Source: CAD feature listing. Evaluate the final solid. Frame: model axes, mm. Coordinates: 2 decimals unless noted, no trailing zeros. Order: outer loops, then holes, each group sorted by start corner. A loop starts at its lowest first (then second) coordinate and runs counter-clockwise, first axis right, second up. Notation, with made-up numbers: (-28.5, 4) - (-16.5, 4) arc R16 ccw to (-16.5, 24) - close; hole circle Ø6 at (20.5, -8). An arc over 180 degrees is marked (long way). One line per question, with ' | ' between items. Start each with the question number.
(1) Section D-D (x = 30). Return the cut outline in (y, z), then the cut area to 3 significant figures.
(2) Section C-C (y = -53). Return the cut outline in (x, z), then the cut area to 3 significant figures.
(3) Section B-B (y = -9). Return the cut outline in (x, z).
(4) Draft query along Y for faces 1 (the cylindrical face through (98.052, -41.158, 0.739)), 2 (the flat face through (58, -37, 0)), 3 (the flat face through (8, -93, 1)), 4 (the flat face through (8, -5, 1)). Return one class per face: +Y half, -Y half, draft (parallel to the pull), parting line (faces both ways), or undercut.
(5) Section A-A (x = 12.5). Return the cut outline in (y, z), then the cut area to 3 significant figures.
(6) Line query: line 1 along Y through (x, z) = (30, 1.1); line 2 along X through (y, z) = (-84, 0.6); line 3 along Y through (x, z) = (36.5, 1.1). Output: solid intervals per line, ascending.
from build123d import *

# Parameters (mm, degrees)
BOSS_EXTRU_1_DEPTH      = 1.5
ESQUISSE2_R             = 1.5
ESQUISSE2_W             = 14
ESQUISSE2_H             = 14
ENL_V_MAT_EXTRU_1_DEPTH = 1.5
D_GAGEMENT_M31_D        = 3.6


with BuildPart() as part:
    # Esquisse1 → Boss.-Extru.1 (new body)
    with BuildSketch(Plane.XY):
        Polygon((0, -85), (16, -101), (117.25, -101), (117.25, 3), (16, 3), (0, -13), align=None)
    extrude(amount=BOSS_EXTRU_1_DEPTH)

    # Esquisse2 → Enlèv. mat.-Extru.1 (cut)
    with BuildSketch(Plane.XY.offset(1.5)):
        with Locations((30, -9)):
            Circle(ESQUISSE2_R)
        with Locations((11, -32.85)):
            Rectangle(ESQUISSE2_W, ESQUISSE2_H)
        with Locations((30.05, -32.85)):
            Rectangle(ESQUISSE2_W, ESQUISSE2_H)
        with Locations((49.1, -32.85)):
            Rectangle(ESQUISSE2_W, ESQUISSE2_H)
        with Locations((68.15, -32.85)):
            Rectangle(ESQUISSE2_W, ESQUISSE2_H)
        with Locations((87.2, -32.85)):
            Rectangle(ESQUISSE2_W, ESQUISSE2_H)
        with Locations((106.25, -32.85)):
            Rectangle(ESQUISSE2_W, ESQUISSE2_H)
        with Locations((30.05, -51.9)):
            Rectangle(ESQUISSE2_W, ESQUISSE2_H)
        with Locations((49.1, -51.9)):
            Rectangle(ESQUISSE2_W, ESQUISSE2_H)
        with Locations((68.15, -51.9)):
            Rectangle(ESQUISSE2_W, ESQUISSE2_H)
        with Locations((87.2, -51.9)):
            Rectangle(ESQUISSE2_W, ESQUISSE2_H)
        with Locations((106.25, -51.9)):
            Rectangle(ESQUISSE2_W, ESQUISSE2_H)
        with Locations((30.05, -70.95)):
            Rectangle(ESQUISSE2_W, ESQUISSE2_H)
        with Locations((49.1, -70.95)):
            Rectangle(ESQUISSE2_W, ESQUISSE2_H)
        with Locations((68.15, -70.95)):
            Rectangle(ESQUISSE2_W, ESQUISSE2_H)
        with Locations((87.2, -70.95)):
            Rectangle(ESQUISSE2_W, ESQUISSE2_H)
        with Locations((106.25, -70.95)):
            Rectangle(ESQUISSE2_W, ESQUISSE2_H)
        with Locations((11, -51.9)):
            Rectangle(ESQUISSE2_W, ESQUISSE2_H)
        with Locations((11, -70.95)):
            Rectangle(ESQUISSE2_W, ESQUISSE2_H)
        with Locations((49.1, -90)):
            Rectangle(ESQUISSE2_W, ESQUISSE2_H)
        with Locations((68.15, -90)):
            Rectangle(ESQUISSE2_W, ESQUISSE2_H)
        with Locations((87.2, -90)):
            Rectangle(ESQUISSE2_W, ESQUISSE2_H)
        with Locations((106.25, -90)):
            Rectangle(ESQUISSE2_W, ESQUISSE2_H)
        with Locations((24.97, -90)):
            Rectangle(ESQUISSE2_W, ESQUISSE2_H)
    extrude(amount=-ENL_V_MAT_EXTRU_1_DEPTH, mode=Mode.SUBTRACT)

    # Dégagement M31 (through all)
    with Locations(Plane.XY.offset(1.5)):
        with Locations((20.525, -42.375), (96.725, -42.375), (96.725, -80.475), (39.575, -80.475)):
            Hole(D_GAGEMENT_M31_D / 2)


solid = part.part
Response values:
1) outline: (-101, 0) - (-97, 0) - (-97, 1.5) - (-101, 1.5) - close; (-83, 0) - (-77.95, 0) - (-77.95, 1.5) - (-83, 1.5) - close; (-63.95, 0) - (-58.9, 0) - (-58.9, 1.5) - (-63.95, 1.5) - close; (-44.9, 0) - (-39.85, 0) - (-39.85, 1.5) - (-44.9, 1.5) - close; (-25.85, 0) - (-10.5, 0) - (-10.5, 1.5) - (-25.85, 1.5) - close; (-7.5, 0) - (3, 0) - (3, 1.5) - (-7.5, 1.5) - close | area: 67.5 mm²
2) outline: (0, 0) - (4, 0) - (4, 1.5) - (0, 1.5) - close; (18, 0) - (23.05, 0) - (23.05, 1.5) - (18, 1.5) - close; (37.05, 0) - (42.1, 0) - (42.1, 1.5) - (37.05, 1.5) - close; (56.1, 0) - (61.15, 0) - (61.15, 1.5) - (56.1, 1.5) - close; (75.15, 0) - (80.2, 0) - (80.2, 1.5) - (75.15, 1.5) - close; (94.2, 0) - (99.25, 0) - (99.25, 1.5) - (94.2, 1.5) - close; (113.25, 0) - (117.25, 0) - (117.25, 1.5) - (113.25, 1.5) - close | area: 49.9 mm²
3) outline: (4, 0) - (28.5, 0) - (28.5, 1.5) - (4, 1.5) - close; (31.5, 0) - (117.25, 0) - (117.25, 1.5) - (31.5, 1.5) - close
4) face 1: undercut | face 2: draft | face 3: -Y half | face 4: +Y half
5) outline: (-97.5, 0) - (-77.95, 0) - (-77.95, 1.5) - (-97.5, 1.5) - close; (-63.95, 0) - (-58.9, 0) - (-58.9, 1.5) - (-63.95, 1.5) - close; (-44.9, 0) - (-39.85, 0) - (-39.85, 1.5) - (-44.9, 1.5) - close; (-25.85, 0) - (-0.5, 0) - (-0.5, 1.5) - (-25.85, 1.5) - close | area: 82.5 mm²
6) line 1: y = -101 to -97, -83 to -77.95, -63.95 to -58.9, -44.9 to -39.85, -25.85 to -10.5, -7.5 to 3 | line 2: x = 0 to 17.97, 31.97 to 42.1, 56.1 to 61.15, 75.15 to 80.2, 94.2 to 99.25, 113.25 to 117.25 | line 3: y = -101 to -77.95, -63.95 to -58.9, -44.9 to -39.85, -25.85 to 3
